```python
from build123d import *

# Parameters (mm, degrees)
F0_R     = 31.75
F0_R_2   = 3.175
F0_R_3   = 15.875
F1_DEPTH = 12.7
F2_DEPTH = 25.4
F3_R     = 9.525
F4_DEPTH = 25.401


with BuildPart() as f1:
    # F0 (on Top) → F1 (new body)
    with BuildSketch(Plane.XY):
        Circle(F0_R)
        with Locations((0, -25.4)):
            Circle(F0_R_2, mode=Mode.SUBTRACT)
        with Locations((-25.4, 0)):
            Circle(F0_R_2, mode=Mode.SUBTRACT)
        Circle(F0_R_3, mode=Mode.SUBTRACT)
        with Locations((25.4, 0)):
            Circle(F0_R_2, mode=Mode.SUBTRACT)
        with Locations((0, 25.4)):
            Circle(F0_R_2, mode=Mode.SUBTRACT)
    extrude(amount=F1_DEPTH)

    # F0 (on Top) → F2 (join)
    with BuildSketch(Plane.XY):
        Circle(F0_R_3)
    extrude(amount=F2_DEPTH)

    # F3 (on face) → F4 (cut, through all)
    with BuildSketch(Plane.XY.offset(25.4)):
        Circle(F3_R)
    extrude(amount=-F4_DEPTH, mode=Mode.SUBTRACT)


solid = f1.part
```
Design review of the part built by this model. Coordinates are the model's own, in mm. A direction names the side the tool comes from. Give positions to 0.01 mm unless a question says otherwise; leave off trailing zeros. Loops run counter-clockwise (first coordinate to the right, second up) from the corner with the lowest first, then second, coordinate; pieces in that order, holes last. Notation, with made-up numbers: (14.25, 77) -> (66.25, 77) arc R16 cw to (66.25, 94) -> close; hole circle Ø6 at (-17, 10). An arc over 180 degrees is marked (long way). Write each question's results on one line, items separated by ' | '.
Q1. Machinability: for faces 1 (the face through (-3.441, -15.497, 18.961)), 2 (the face through (7, -7, 25.4)), which of the approach directions +Z, -Z, +X, -X, +Y, -Y give a long, thin tool a straight path to every point of the face, cutting with its end or side? Answer none if there is none.
Reply:
face 1: +Z | face 2: +Z, +X, -X, +Y, -Y
Q2. Wall thickness on L1, parallel to Y at x = 0, z = 10.25 (3 decimals); L2, parallel to Z at x = 3.5, y = 19; L3, parallel to Y at x = 4.5, z = 10: over which ranges is each line inside the solid? List them lowest first.
Reply:
L1: y = -31.75 to -28.575, -22.225 to -9.525, 9.525 to 22.225, 28.575 to 31.75 | L2: z = 0 to 12.7 | L3: y = -31.43 to -8.39, 8.39 to 31.43
Q3. Take a section at C-C, the plane z = 10.25. Write out the cut boundary in (x, y) (3 decimals), plus the area to 3 significant figures.
Reply:
outline: circle Ø63.5 at (0, 0); hole circle Ø6.35 at (-25.4, 0); hole circle Ø19.05 at (0, 0); hole circle Ø6.35 at (0, -25.4); hole circle Ø6.35 at (0, 25.4); hole circle Ø6.35 at (25.4, 0) | area: 2,760 mm²
Q4. Take a section at D-D, the plane x = -11.5. Write out the cut boundary in (y, z).
Reply:
outline: (-29.59, 0) -> (29.59, 0) -> (29.59, 12.7) -> (10.94, 12.7) -> (10.94, 25.4) -> (-10.94, 25.4) -> (-10.94, 12.7) -> (-29.59, 12.7) -> close
Q5. Take a section at A-A, the plane y = 25.4. Write out the cut boundary in (x, z) (3 decimals).
Reply:
outline: (-19.05, 0) -> (-3.175, 0) -> (-3.175, 12.7) -> (-19.05, 12.7) -> close; (3.175, 0) -> (19.05, 0) -> (19.05, 12.7) -> (3.175, 12.7) -> close
Q6. For pin 1 Ø4 at (x, z) = (15, 17.5) entering from +Y; pin 2 Ø10 at (x, z) = (-16.5, 11) entering from +Y; pin 3 Ø10 at (x, y) = (-0.5, 9.5) entering from -Z; pin 4 Ø4 at (y, z) = (14, 21) entering from -X, all flat-tipped, find the tip position at first contact; note any pin that passes through.
Reply:
pin 1: stops at y = 9.11 | pin 2: stops at y = 29.59 | pin 3: stops at z = 0 | pin 4: stops at x = -10.39
Q7. The part is to be moulded in two halves that separate along X. For faces 3 (the face through (7, 15, 12.7)), 4 (the face through (-0.41, -22.25, 6.26)), 5 (the face through (-0.41, 28.55, 6.26)), 6 (the face through (-6.883, -30.995, 6.261)), say which applies: +X half, -X half, draft (parallel to the pull), parting line (faces both ways), or undercut.
Reply:
face 3: draft | face 4: undercut | face 5: undercut | face 6: parting line
